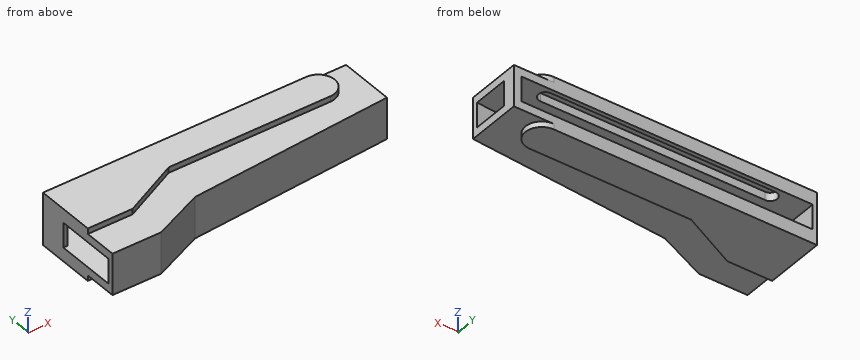
```python
from build123d import *

# Parameters (mm, degrees)
BOSS_EXTRUDE1_START = 3
BOSS_EXTRUDE1_DEPTH = 1.5
BOSS_EXTRUDE2_DEPTH = 1
CUT_EXTRUDE1_DEPTH  = 1.5
BOSS_EXTRUDE3_START = -3
BOSS_EXTRUDE3_DEPTH = 1.5
BOSS_EXTRUDE4_DEPTH = 1
BOSS_EXTRUDE5_DEPTH = 4.5
CUT_EXTRUDE2_DEPTH  = 1
SKETCH10_W          = 0.780201508
SKETCH10_H          = 4.986255627
BOSS_EXTRUDE6_DEPTH = 4.5
SKETCH11_W          = 1.426663005
SKETCH11_H          = 2.471476461
BOSS_EXTRUDE7_DEPTH = 4.5


with BuildPart() as part:
    # Sketch1 → Boss-Extrude1 (new body)
    with BuildSketch(Plane.XY.offset(BOSS_EXTRUDE1_START)):
        Polygon((-9.513255025, -4.466723996), (-18.663811547, -8.5), (-27.5, -8.5), (-27.5, 8.5), (27.5, 8.5), (27.5, -1.5), align=None)
    extrude(amount=BOSS_EXTRUDE1_DEPTH)

    # Sketch2 → Boss-Extrude2 (add)
    with BuildSketch(Plane.XY.offset(4.5)):
        with BuildLine():
            Line((-27.5, -2.468678655), (-19.36276873, -2.468678655))
            Line((-19.36276873, -2.468678655), (-9.07165048, 2.587651121))
            Line((-9.07165048, 2.587651121), (20.25506222, 2.587651121))
            ThreePointArc((20.25506222, 2.587651121), (23.21123666, 5.54382556), (20.25506222, 8.5))
            Line((20.25506222, 8.5), (-27.5, 8.5))
            Line((-27.5, 8.5), (-27.5, -2.468678655))
        make_face()
    extrude(amount=BOSS_EXTRUDE2_DEPTH)

    # Sketch3 → Cut-Extrude1 (cut)
    with BuildSketch(Plane(origin=(0, 0, 3), x_dir=(-1, 0, 0), z_dir=(0, 0, -1))):
        with BuildLine():
            Line((-20.296822584, 7.75), (20.5, 7.75))
            ThreePointArc((20.5, 7.75), (21.75, 6.5), (20.5, 5.25))
            Line((20.5, 5.25), (-20.296822584, 5.25))
            ThreePointArc((-20.296822584, 5.25), (-21.546822584, 6.5), (-20.296822584, 7.75))
        make_face()
    extrude(amount=-CUT_EXTRUDE1_DEPTH, mode=Mode.SUBTRACT)



with BuildPart() as body_2:
    # Sketch5 → Boss-Extrude3 (new body)
    with BuildSketch(Plane.XY.offset(BOSS_EXTRUDE3_START)):
        Polygon((27.5, -1.5), (-9.513255025, -4.466723996), (-18.663811547, -8.5), (-27.5, -8.5), (-27.5, 8.5), (27.5, 8.5), align=None)
    extrude(amount=BOSS_EXTRUDE3_DEPTH)

    # Sketch7 → Boss-Extrude4 (add)
    with BuildSketch(Plane(origin=(0, 0, -3), x_dir=(-1, 0, 0), z_dir=(0, 0, -1))):
        with BuildLine():
            Line((-20.25506222, 8.5), (27.5, 8.5))
            Line((27.5, 8.5), (27.5, -2.468678655))
            Line((27.5, -2.468678655), (19.36276873, -2.468678655))
            Line((19.36276873, -2.468678655), (9.07165048, 2.587651121))
            Line((9.07165048, 2.587651121), (-20.25506222, 2.587651121))
            ThreePointArc((-20.25506222, 2.587651121), (-23.21123666, 5.54382556), (-20.25506222, 8.5))
        make_face()
    extrude(amount=BOSS_EXTRUDE4_DEPTH)


with BuildPart() as part_1:
    add(part.part)

    add(body_2.part)  # Boss-Extrude5 merges body 2
    # Sketch8 → Boss-Extrude5 (add)
    with BuildSketch(Plane(origin=(0, 0, 3), x_dir=(-1, 0, 0), z_dir=(0, 0, -1))):
        Polygon((-27.5, -0.503196857), (-27.5, -1.5), (9.513255025, -4.466723996), (18.663811547, -8.5), (27.5, -8.5), (27.5, -7.5), (26.5, -7.5), (18.874420362, -7.5), (9.761781861, -3.483437061), (-27.420103222, -0.503196857), align=None)
    extrude(amount=BOSS_EXTRUDE5_DEPTH)

    # Sketch9 → Cut-Extrude2 (cut)
    with BuildSketch(Plane.XY.offset(-1.5)):
        with BuildLine():
            Line((-20.5, 7.75), (20.296822584, 7.75))
            ThreePointArc((20.296822584, 7.75), (21.546822584, 6.5), (20.296822584, 5.25))
            Line((20.296822584, 5.25), (-20.5, 5.25))
            ThreePointArc((-20.5, 5.25), (-21.75, 6.5), (-20.5, 7.75))
        make_face()
    extrude(amount=-CUT_EXTRUDE2_DEPTH, mode=Mode.SUBTRACT)

    # Sketch10 → Boss-Extrude6 (add)
    with BuildSketch(Plane(origin=(0, 0, 3), x_dir=(-1, 0, 0), z_dir=(0, 0, -1))):
        with Locations((27.109899246, 6.006872186)):
            Rectangle(SKETCH10_W, SKETCH10_H)
    extrude(amount=BOSS_EXTRUDE6_DEPTH)

    # Sketch11 → Boss-Extrude7 (add)
    with BuildSketch(Plane.XY.offset(-1.5)):
        with Locations((26.786668498, 7.26426177)):
            Rectangle(SKETCH11_W, SKETCH11_H)
    extrude(amount=BOSS_EXTRUDE7_DEPTH)


solid = part_1.part
```
Check sheet for the modelled part. Datum: model origin and axes. Units: mm. Coordinates: 2 decimals unless noted, no trailing zeros. Write each loop counter-clockwise with the first axis right and the second up, starting at its lowest first coordinate (ties: lowest second). Pieces come first, ordered by that corner, then holes. Notation, with made-up numbers: (57.5, 31.25) -> (116.5, 31.25) arc R16 cw to (116.5, 53.25) -> close; hole circle Ø2 at (73, 60.5). An arc over 180 degrees is marked (long way). Use a Markdown table: item, result.
1. Sectioned sample at C-C (x = -2). Enter the section's corners in (y, z).
Reported:
| item | result |
|---|---|
| outline | (-3.86, -3) -> (2.59, -3) -> (2.59, -4) -> (8.5, -4) -> (8.5, -1.5) -> (7.75, -1.5) -> (7.75, -2.5) -> (5.25, -2.5) -> (5.25, -1.5) -> (-2.86, -1.5) -> (-2.86, 3) -> (5.25, 3) -> (5.25, 4.5) -> (7.75, 4.5) -> (7.75, 3) -> (8.5, 3) -> (8.5, 5.5) -> (2.59, 5.5) -> (2.59, 4.5) -> (-3.86, 4.5) -> close |
2. Scan lines: line 1 along Z through (x, y) = (-23.5, -2.25); line 2 along Z through (x, y) = (-6, 6.5); line 3 along X through (y, z) = (6.25, 0.5). Record each from-to range of solid material in increasing order.
Reported:
| item | result |
|---|---|
| line 1 | z = -4 to -1.5, 3 to 5.5 |
| line 2 | z = -4 to -2.5, 4.5 to 5.5 |
| line 3 | x = -27.5 to -26.72, 26.07 to 27.5 |
3. Sectioned sample at A-A (z = 1.25). Enter the section's corners in (x, y).
Reported:
| item | result |
|---|---|
| outline | (-27.5, -8.5) -> (-18.66, -8.5) -> (-9.51, -4.47) -> (27.5, -1.5) -> (27.5, -0.5) -> (27.42, -0.5) -> (-9.76, -3.48) -> (-18.87, -7.5) -> (-27.5, -7.5) -> close; (-27.5, 3.51) -> (-26.72, 3.51) -> (-26.72, 8.5) -> (-27.5, 8.5) -> close; (26.07, 6.03) -> (27.5, 6.03) -> (27.5, 8.5) -> (26.07, 8.5) -> close |
4. Sectioned sample at B-B (y = 0). Enter the section's corners in (x, z), plus the area to 3 significant figures.
Reported:
| item | result |
|---|---|
| outline | (-27.5, -4) -> (-14.34, -4) -> (-14.34, -3) -> (27.5, -3) -> (27.5, -1.5) -> (-27.5, -1.5) -> close; (-27.5, 3) -> (27.5, 3) -> (27.5, 4.5) -> (-14.34, 4.5) -> (-14.34, 5.5) -> (-27.5, 5.5) -> close |
| area | 191 mm2 |
5. Go/stop test with flat-tipped pins: pin 1 Ø1.5 at (x, z) = (-14.5, 3) entering from -Y; pin 2 Ø1.5 at (x, z) = (3, 1.5) entering from -Y; pin 3 Ø1.1 at (x, z) = (11.5, -3.5) entering from -Y; pin 4 Ø3.5 at (x, z) = (-24.5, 1.5) entering from +Y. Record where each tip stops, or that it passes through.
Reported:
| item | result |
|---|---|
| pin 1 | stops at y = -7 |
| pin 2 | stops at y = -3.52 |
| pin 3 | stops at y = -2.8 |
| pin 4 | stops at y = 8.5 |
6. Sectioned sample at D-D (y = 6.5). Enter the section's corners in (x, z), plus the area to 3 significant figures.
Reported:
| item | result |
|---|---|
| outline | (-27.5, -4) -> (23.05, -4) -> (23.05, -3) -> (27.5, -3) -> (27.5, 4.5) -> (23.05, 4.5) -> (23.05, 5.5) -> (-27.5, 5.5) -> close; hole (-26.72, -1.5) -> (-21.75, -1.5) -> (-21.75, -2.5) -> (21.55, -2.5) -> (21.55, -1.5) -> (26.07, -1.5) -> (26.07, 3) -> (21.55, 3) -> (21.55, 4.5) -> (-21.75, 4.5) -> (-21.75, 3) -> (-26.72, 3) -> close |
| area | 168 mm2 |
